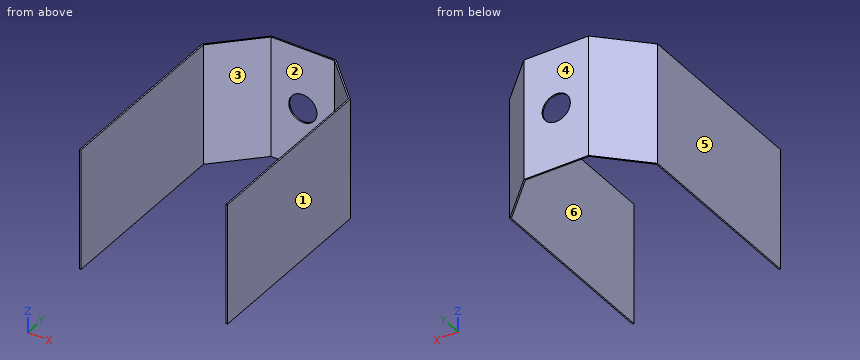
from build123d import *

# Parameters (mm, degrees)
EXTRUDE_1_DEPTH     = 171.62
SKETCH_2_R          = 20
CUT_EXTRUDE_1_DEPTH = 384.382537519


with BuildPart() as part:
    # Эскиз1 → Вытянуть-Тонкостенный1 (new body)
    with BuildSketch(Plane.XY):
        Polygon((-96.72523491, 314.926453532), (-96.72523491, 579.392619017), (-37.621355545, 638.496497272), (54.170886835, 638.496497272), (113.274765367, 579.39261874), (113.27476147, 314.926454672), (111.27476147, 314.926454702), (111.274765355, 578.564191627), (53.34245971, 636.496497272), (-36.792928431, 636.496497272), (-94.72523491, 578.564191882), (-94.72523491, 314.926453532), align=None)
    extrude(amount=EXTRUDE_1_DEPTH)

    # Эскиз2 → Вырез-Вытянуть1 (cut, through all)
    with BuildSketch(Plane(origin=(0, 638.496497272, 0), x_dir=(1, 0, 0), z_dir=(0, 1, 0))):
        with Locations(Location((8.274765645, -85.81, 0), (0, 0, 270))):
            Circle(SKETCH_2_R)
    extrude(amount=-CUT_EXTRUDE_1_DEPTH, mode=Mode.SUBTRACT)


solid = part.part
Design review of the part built by this model. Coordinates are the model's own, in mm. Face numbers are marked on the shaded views. A direction names the side the tool comes from. Give positions to 0.01 mm unless a question says otherwise; leave off trailing zeros. Write each loop counter-clockwise with the first axis right and the second up, starting at its lowest first coordinate (ties: lowest second). Pieces come first, ordered by that corner, then holes. Notation, with made-up numbers: M 45,-32 L 58,-32 A26 ccw 58,-12 Z; hole C -40,-38.5 d6. An arc over 180 degrees is marked long. Answer as a JSON object with one key per item and string values. Group by question number.
1) For line 1 along X through (y, z) = (540.5, 94.5); line 2 along Y through (x, z) = (-31.5, 48.5); line 3 along X through (y, z) = (637, 85), list the stretches that pass through material, from the lowest coordinate up.
2) We need section C-C (x = 12). Give the boundary of the cut face in (y, z).
3) Tool access review of the marked faces 5 and 6: name each direction out of +Z, -Z, +X, -X, +Y, -Y from which nothing blocks a thin tool from reaching the whole face with its end or side.
4) We need section D-D (z = 31). Give the boundary of the cut face in (x, y), and give its area (3 significant figures).
5) We need section B-B (z = 85.81). Give the boundary of the cut face in (x, y).
6) Clearance check with flat-ended pins moving along their axes: pin 1 Ø1.5 at (x, z) = (78, 59) entering from +Y; pin 2 Ø24 at (x, z) = (8.27, 85.81) entering from -Y (1 decimal); pin 3 Ø2 at (x, z) = (13.5, 50) entering from -Y. State where each tip first meets the part, or that it passes through.
7) We need section A-A (y = 543). Give the boundary of the cut face in (x, z), and give its area (3 significant figures).
8) Mouldability with a two-part tool opening along X and no side actions: class the marked faces 1, 2, 3 and 4 as released by +X, released by -X, zero draft, split by the parting line, or undercut.
Answer key:
{
 "1": {"line 1": "x = -96.73 to -94.73, 111.27 to 113.27", "line 2": "y = 636.5 to 638.5", "line 3": "x = -39.12 to -11.71, 28.26 to 55.67"},
 "2": {"outline": "M 636.5,0 L 638.5,0 L 638.5,66.16 L 636.5,66.16 Z; M 636.5,105.46 L 638.5,105.46 L 638.5,171.62 L 636.5,171.62 Z"},
 "3": {"face 5": "+Z, -Z, -X, +Y, -Y", "face 6": "+Z, -Z, -Y"},
 "4": {"outline": "M -96.73,314.93 L -94.73,314.93 L -94.73,578.56 L -36.79,636.5 L 53.34,636.5 L 111.27,578.56 L 111.27,314.93 L 113.27,314.93 L 113.27,579.39 L 54.17,638.5 L -37.62,638.5 L -96.73,579.39 Z", "area": "1,570 mm²"},
 "5": {"outline": "M -96.73,314.93 L -94.73,314.93 L -94.73,578.56 L -36.79,636.5 L -11.73,636.5 L -11.73,638.5 L -37.62,638.5 L -96.73,579.39 Z; M 28.27,636.5 L 53.34,636.5 L 111.27,578.56 L 111.27,314.93 L 113.27,314.93 L 113.27,579.39 L 54.17,638.5 L 28.27,638.5 Z"},
 "6": {"pin 1": "stops at y = 615.42", "pin 2": "passes through", "pin 3": "stops at y = 636.5"},
 "7": {"outline": "M -96.73,0 L -94.73,0 L -94.73,171.62 L -96.73,171.62 Z; M 111.27,0 L 113.27,0 L 113.27,171.62 L 111.27,171.62 Z", "area": "686 mm²"},
 "8": {"face 1": "released by +X", "face 2": "undercut", "face 3": "undercut", "face 4": "zero draft"}
}
